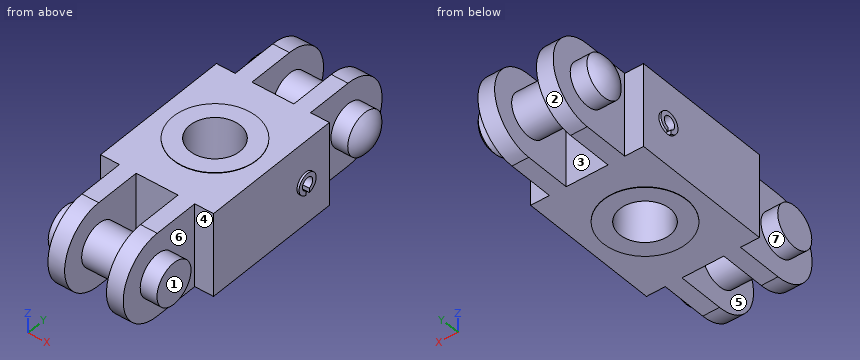
from build123d import *

# Parameters (mm, degrees)
ESQUISSE1_R          = 10
BASE_EXTRUSION_DEPTH = 10
ESQUISSE2_OUTSIDE_W  = 38.62
ESQUISSE2_OUTSIDE_H  = 94.62
D_TOURAGE_DEPTH      = 48.675989764
ESQUISSE3_R          = 5
AL_SAGES_DEPTH       = 46.279686395
ESQUISSE4_R          = 5
AXES_DEPTH           = 13
ESQUISSE5_R          = 10
ESQUISSE5_R_2        = 6
ECROU_RAPPORT_DEPTH  = 10.1
ESQUISSE6_R          = 2.5
PER_AGE_DEPTH        = 49.561919237
GOUPILLE_DEPTH       = 14


# Read off the part's stored shape, not the designer's step: Dôme1, Dôme2
with BuildPart() as part:
    # Esquisse1 → Base-Extrusion (new, symmetric)
    with BuildSketch(Plane.XY):
        Polygon((-13.5, -17), (-13.5, 17), (-9, 17), (-9, 38), (-5, 38), (-5, 17), (5, 17), (5, 38), (9, 38), (9, 17), (13.5, 17), (13.5, -17), (9, -17), (9, -38), (5, -38), (5, -17), (-5, -17), (-5, -38), (-9, -38), (-9, -17), align=None)
        Circle(ESQUISSE1_R, mode=Mode.SUBTRACT)
    extrude(amount=BASE_EXTRUSION_DEPTH, both=True)

    # Esquisse2 outside → Détourage (cut, through all)
    with BuildSketch(Plane.ZY.offset(13.5)):
        Rectangle(ESQUISSE2_OUTSIDE_W, ESQUISSE2_OUTSIDE_H)
        with BuildLine():
            Line((-10, 28), (-10, -28))
            ThreePointArc((-10, -28), (0, -38), (10, -28))
            Line((10, -28), (10, 28))
            ThreePointArc((10, 28), (0, 38), (-10, 28))
        make_face(mode=Mode.SUBTRACT)
    extrude(amount=-D_TOURAGE_DEPTH, mode=Mode.SUBTRACT)

    # Esquisse3 → Alésages (cut, through all)
    with BuildSketch(Plane.ZY.offset(9)):
        with Locations(Location((0, 28, 0), (0, 0, 270))):
            Circle(ESQUISSE3_R)
        with Locations(Location((0, -28, 0), (0, 0, 270))):
            Circle(ESQUISSE3_R)
    extrude(amount=-AL_SAGES_DEPTH, mode=Mode.SUBTRACT)

    # Esquisse4 → Axes (add, symmetric)
    with BuildSketch(Plane(origin=(0, 0, 0), x_dir=(0, 0, -1), z_dir=(1, 0, 0))):
        with Locations(Location((0, -28, 0), (0, 0, 180))):
            Circle(ESQUISSE4_R)
        with Locations(Location((0, 28, 0), (0, 0, 180))):
            Circle(ESQUISSE4_R)
    extrude(amount=AXES_DEPTH, both=True)

    # Dôme1 outline → Dôme1 (revolve)
    with BuildSketch(Plane(origin=(0, 28, 0), x_dir=(0, 1, 0), z_dir=(0, 0, -1))):
        with BuildLine():
            Line((0, 13), (5.000000005, 12.999999995))
            ThreePointArc((5.000000005, 12.999999995), (2.692582407, 14.481456008), (0, 15))
            Line((0, 15), (0, 13))
        make_face()
    revolve(axis=Axis((0, 28, 0), (1, 0, 0)))

    # Dôme2 outline → Dôme2 (revolve)
    with BuildSketch(Plane(origin=(0, 28, 0), x_dir=(0, 1, 0), z_dir=(0, 0, -1))):
        with BuildLine():
            Line((0, -12.999999995), (0, -15))
            ThreePointArc((0, -15), (2.692582407, -14.481456008), (5.000000005, -12.999999995))
            Line((5.000000005, -12.999999995), (0, -12.999999995))
        make_face()
    revolve(axis=Axis((0, 28, 0), (1, 0, 0)))

    # Esquisse5 → Ecrou rapporté (add, symmetric)
    with BuildSketch(Plane.XY):
        Circle(ESQUISSE5_R)
        Circle(ESQUISSE5_R_2, mode=Mode.SUBTRACT)
    extrude(amount=ECROU_RAPPORT_DEPTH, both=True)

    # Esquisse6 → Perçage (cut, through all)
    with BuildSketch(Plane(origin=(13.5, 0, 0), x_dir=(0, 0, -1), z_dir=(1, 0, 0))):
        with Locations((0, 10)):
            Circle(ESQUISSE6_R)
    extrude(amount=-PER_AGE_DEPTH, mode=Mode.SUBTRACT)

    # Esquisse7 → Goupille (add, symmetric)
    with BuildSketch(Plane(origin=(0, 0, 0), x_dir=(0, 0, -1), z_dir=(1, 0, 0))):
        with BuildLine():
            Line((1.414213562, 10.5), (2.449489743, 10.5))
            ThreePointArc((2.449489743, 10.5), (-2.5, 10), (2.449489743, 9.5))
            Line((2.449489743, 9.5), (1.414213562, 9.5))
            ThreePointArc((1.414213562, 9.5), (-1.5, 10), (1.414213562, 10.5))
        make_face()
    extrude(amount=GOUPILLE_DEPTH, both=True)


solid = part.part
Here's how the part is built. I have some questions about the finished solid (model axes, mm). Face numbers are marked on the shaded views. A direction names the side the tool comes from. Round coordinates to 2 decimals unless told otherwise and drop trailing zeros. Loops run counter-clockwise (first coordinate to the right, second up) from the corner with the lowest first, then second, coordinate; pieces in that order, holes last. Notation, with made-up numbers: M 28.25,0 L 42.25,0 A29 ccw 42.25,30 Z; hole C 56,77 d9. An arc over 180 degrees is marked long. Write each question's results on one line, items separated by ' | '. Start each with the question number.
(1) I want a section at B-B (y = 0). Please give me the cut outline in (x, z), then the cut area to 3 significant figures.
(2) I want a section at C-C (z = 0). State how many separate pieces and enclosed holes the cut face has, then the cut area to 3 significant figures.
(3) On a 3-axis mill with a long thin cutter (end or side, diameter ignored), from which of +Z, -Z, +X, -X, +Y, -Y can I reach the whole of each face in a straight line? I mean the marked faces 4, 5, 6 and 7. Say none if no direction works.
(4) Thinking about a two-plate mould opening in Y: for the marked faces 1, 2 and 3, which applies, pulls with the +Y half, pulls with the -Y half, needs draft (parallel to the pull), parting line crosses it, or undercut?
(5) If I drill on probe 1 along X at (y, z) = (21, 5.75); probe 2 along Y at (x, z) = (0.5, 0); probe 3 along Y at (x, z) = (-8, 0), over which ranges is the centre line in solid material (lowest first)? Write a range as from..to.
(6) I want a section at D-D (z = 8.5). Please give me the cut outline in (x, y), then the cut area to 3 significant figures.
(7) I want a section at A-A (x = 0). Please give me the cut outline in (y, z), then the cut area to 3 significant figures.
(8) Will these pins go through, and if not, where does the flat tip stop? P1, Ø12, axis at y = 3, z = 7.5, coming from the -X side; P2, Ø1.5, axis at x = 2, y = 16, coming from the -Z side; P3, Ø5.5, axis at y = 10, z = 0, coming from the +X side.
Solved:
1) outline: M -13.5,-10 L -10,-10 L -10,-10.1 L -6,-10.1 L -6,10.1 L -10,10.1 L -10,10 L -13.5,10 Z; M 6,-10.1 L 10,-10.1 L 10,-10 L 13.5,-10 L 13.5,10 L 10,10 L 10,10.1 L 6,10.1 Z | area: 302 mm²
2) separate pieces: 2 | enclosed holes: 3 | area: 1,450 mm²
3) face 4: +Z, -Z, +X | face 5: none | face 6: +X | face 7: -X
4) face 1: needs draft | face 2: pulls with the +Y half | face 3: undercut
5) probe 1: x = -9..-5, 5..9 | probe 2: y = -33..-23, -17..-5.98, 5.98..8.5, 11.5..17, 23..33 | probe 3: y = -38..8.5, 11.5..38
6) outline: M -13.5,-17 L -9,-17 L -9,-33.27 L -5,-33.27 L -5,-17 L 5,-17 L 5,-33.27 L 9,-33.27 L 9,-17 L 13.5,-17 L 13.5,17 L 9,17 L 9,33.27 L 5,33.27 L 5,17 L -5,17 L -5,33.27 L -9,33.27 L -9,17 L -13.5,17 Z; hole C 0,0 d12 | area: 1,070 mm²
7) outline: C -28,0 d10; M -17,-10 L -10,-10 L -10,-10.1 L -6,-10.1 L -6,10.1 L -10,10.1 L -10,10 L -17,10 Z; M 6,-10.1 L 10,-10.1 L 10,-10 L 17,-10 L 17,10 L 10,10 L 10,10.1 L 6,10.1 Z; C 28,0 d10; hole M 9.5,-2.45 A2.5 ccw 10.5,-2.45 L 10.5,-1.41 A1.5 ccw long 9.5,-1.41 Z | area: 591 mm²
8) P1: stops at x = -13.5 | P2: stops at z = -10 | P3: stops at x = 14
